Can you work these out from the model? Positions are in its coordinate system, mm. Coordinates: 2 decimals unless noted, no trailing zeros. Loops run counter-clockwise (first coordinate to the right, second up) from the corner with the lowest first, then second, coordinate; pieces in that order, holes last. Notation, with made-up numbers: (25.25, 3) -> (58.25, 3) arc R36 cw to (58.25, 39) -> close; hole circle Ø11 at (71.25, 24.25). An arc over 180 degrees is marked (long way). Put each result on its own line as item: value. Start each with the question number.
Item 1: If we section it at B-B on x = 15: Please give me the cut outline in (y, z), plus the area to 3 significant figures.
Item 2: We'd pull the mould along Z, two halves only. Please class faces 1 (the flat face through (-25, 6, 0)), 2 (the flat face through (0, 6, 25)), 3 (the cylindrical face through (-12.918, 6.591, 4.727)): pulls with the +Z half, pulls with the -Z half, needs draft (parallel to the pull), parting line crosses it, or undercut.
Item 3: Please list where these lines run through material, in increasing order: L1, parallel to X at y = 7.5, z = 5; L2, parallel to X at y = 1, z = 5.5. Write a range as from..to.
Item 4: Will these pins go through, and if not, where does the flat tip stop? P1, Ø2.5, axis at x = 15, z = 5, coming from the +Y side; P2, Ø12, axis at x = 16.5, z = -5.5, coming from the -Y side.
Item 5: If we section it at A-A on z = 5: Please give me the cut outline in (x, y).
```python
from build123d import *

# Parameters (mm, degrees)
SKETCH_1_W          = 50
SKETCH_1_H          = 50
EXTRUDE_1_DEPTH     = 13
CUT_EXTRUDE_1_REACH = 39.67
SKETCH_3_R          = 2.1


with BuildPart() as part:
    # 草图1 → 凸台-拉伸1 (new body)
    with BuildSketch(Plane(origin=(0, 0, 0), x_dir=(1, 0, 0), z_dir=(0, 1, 0))):
        Rectangle(SKETCH_1_W, SKETCH_1_H)
    extrude(amount=EXTRUDE_1_DEPTH)

    # 草图3 → 切除-拉伸1 (cut, up to next)
    with BuildSketch(Plane(origin=(0, 13, 0), x_dir=(1, 0, 0), z_dir=(0, 1, 0)), mode=Mode.PRIVATE) as cut_extrude_1_sk1:
        with Locations(Location((-15, -5, 0), (0, 0, 270))):
            Circle(SKETCH_3_R)
    cut_extrude_1_tool1 = extrude(cut_extrude_1_sk1.sketch, amount=-CUT_EXTRUDE_1_REACH, mode=Mode.PRIVATE) & part.part
    # 草图3 → 切除-拉伸1 (cut, up to next)
    with BuildSketch(Plane(origin=(0, 13, 0), x_dir=(1, 0, 0), z_dir=(0, 1, 0)), mode=Mode.PRIVATE) as cut_extrude_1_sk2:
        with Locations(Location((15, -5, 0), (0, 0, 270))):
            Circle(SKETCH_3_R)
    cut_extrude_1_tool2 = extrude(cut_extrude_1_sk2.sketch, amount=-CUT_EXTRUDE_1_REACH, mode=Mode.PRIVATE) & part.part
    add(cut_extrude_1_tool1.solids().sort_by_distance((-15, 13, 5))[0], mode=Mode.SUBTRACT)
    add(cut_extrude_1_tool2.solids().sort_by_distance((15, 13, 5))[0], mode=Mode.SUBTRACT)


solid = part.part
```
Solutions:
1. outline: (0, -25) -> (13, -25) -> (13, 2.9) -> (0, 2.9) -> close; (0, 7.1) -> (13, 7.1) -> (13, 25) -> (0, 25) -> close
1. area: 595 mm^2
2. face 1: needs draft
2. face 2: pulls with the +Z half
2. face 3: undercut
3. L1: -25..-17.1, -12.9..12.9, 17.1..25
3. L2: -25..-17.04, -12.96..12.96, 17.04..25
4. P1: through
4. P2: y = 0
5. outline: (-25, 0) -> (-17.1, 0) -> (-17.1, 13) -> (-25, 13) -> close; (-12.9, 0) -> (12.9, 0) -> (12.9, 13) -> (-12.9, 13) -> close; (17.1, 0) -> (25, 0) -> (25, 13) -> (17.1, 13) -> close
